Geometry check sheet. Reference: the model listing, model coordinates, mm. Face numbers are marked on the shaded views. Round coordinates to 2 decimals unless told otherwise and drop trailing zeros. Order: outer loops, then holes, each group sorted by start corner. A loop starts at its lowest first (then second) coordinate and runs counter-clockwise, first axis right, second up. Notation, with made-up numbers: (-22.5, 21.25) - (10.5, 21.25) arc R14 cw to (10.5, 28.25) - close; hole circle Ø10 at (56, 10). An arc over 180 degrees is marked (long way). Write each question's results on one line, items separated by ' | '.
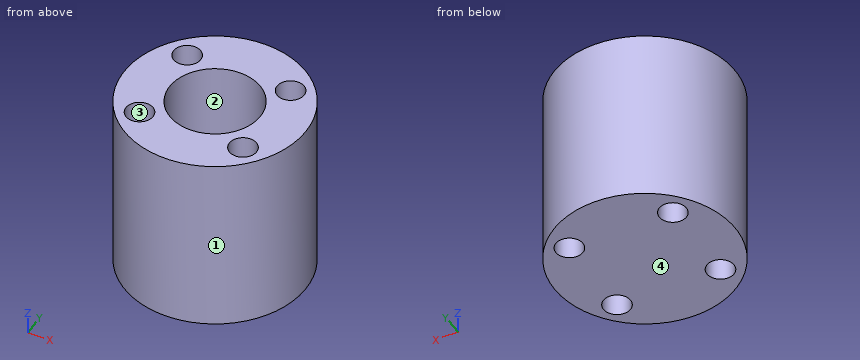
```python
from build123d import *

# Parameters (mm, degrees)
F0_R     = 12.7
F0_R_2   = 1.905
F0_R_3   = 6.35
F1_DEPTH = 25.4
F0_R_4   = 4.0005
F2_DEPTH = 7.62
F3_DEPTH = 7.62


with BuildPart() as f1:
    # F0 (on Top) → F1 (new body)
    with BuildSketch(Plane.XY):
        Circle(F0_R)
        with Locations((-7.286887, -6.266722)):
            Circle(F0_R_2, mode=Mode.SUBTRACT)
        Circle(F0_R_3, mode=Mode.SUBTRACT)
        with Locations((7.286887, -6.266722)):
            Circle(F0_R_2, mode=Mode.SUBTRACT)
        with Locations((-7.286887, 6.266722)):
            Circle(F0_R_2, mode=Mode.SUBTRACT)
        with Locations((7.286887, 6.266722)):
            Circle(F0_R_2, mode=Mode.SUBTRACT)
    extrude(amount=F1_DEPTH)

    # F0 (on Top) → F2 (join)
    with BuildSketch(Plane.XY):
        Circle(F0_R_3)
        Circle(F0_R_4, mode=Mode.SUBTRACT)
    extrude(amount=F2_DEPTH)

    # F0 (on Top) → F3 (join)
    with BuildSketch(Plane.XY):
        Circle(F0_R_4)
    extrude(amount=F3_DEPTH)


solid = f1.part
```
(1) Section check D-D (z = 20.5). Record the cut outline in (x, y) (3 decimals).
Answers follow:
outline: circle Ø25.4 at (0, 0); hole circle Ø3.81 at (-7.287, -6.267); hole circle Ø3.81 at (-7.287, 6.267); hole circle Ø12.7 at (0, 0); hole circle Ø3.81 at (7.287, -6.267); hole circle Ø3.81 at (7.287, 6.267)
(2) Section check A-A (x = 6.75). Record the cut outline in (y, z), then the cut area to 3 significant figures.
Answers follow:
outline: (-10.76, 0) - (-8.09, 0) - (-8.09, 25.4) - (-10.76, 25.4) - close; (-4.44, 0) - (4.44, 0) - (4.44, 25.4) - (-4.44, 25.4) - close; (8.09, 0) - (10.76, 0) - (10.76, 25.4) - (8.09, 25.4) - close | area: 361 mm²
(3) Material ranges on line 1 (Y direction, x = 0, z = 20.75); line 2 (X direction, y = -5.75, z = 15.5); line 3 (Y direction, x = -7.75, z = 10.75), recorded low to high.
Answers follow:
line 1: -12.7 to -6.35, 6.35 to 12.7 | line 2: -11.32 to -9.12, -5.45 to -2.69, 2.69 to 5.45, 9.12 to 11.32 | line 3: -10.06 to -8.11, -4.42 to 4.42, 8.11 to 10.06
(4) Depth check by flat-ended pin: pin 1 Ø3 at (x, z) = (-6.5, 12.5) entering from +Y; pin 2 Ø3 at (x, z) = (9.5, 6.5) entering from +Y; pin 3 Ø5 at (y, z) = (-9.5, 10) entering from -X. Enter the tip coordinate at first touch or a pass-through.
Answers follow:
pin 1: y = 11.67 | pin 2: y = 9.86 | pin 3: x = -10.6
(5) Section check B-B (y = 0). Record the cut outline in (x, z), then the cut area to 3 significant figures.
Answers follow:
outline: (-12.7, 0) - (12.7, 0) - (12.7, 25.4) - (6.35, 25.4) - (6.35, 7.62) - (-6.35, 7.62) - (-6.35, 25.4) - (-12.7, 25.4) - close | area: 419 mm²
(6) Draft check along X on the marked faces 1, 2, 3 and 4. Enter one of: released by +X, released by -X, zero draft, split by the parting line, or undercut.
Answers follow:
face 1: split by the parting line | face 2: undercut | face 3: undercut | face 4: zero draft
